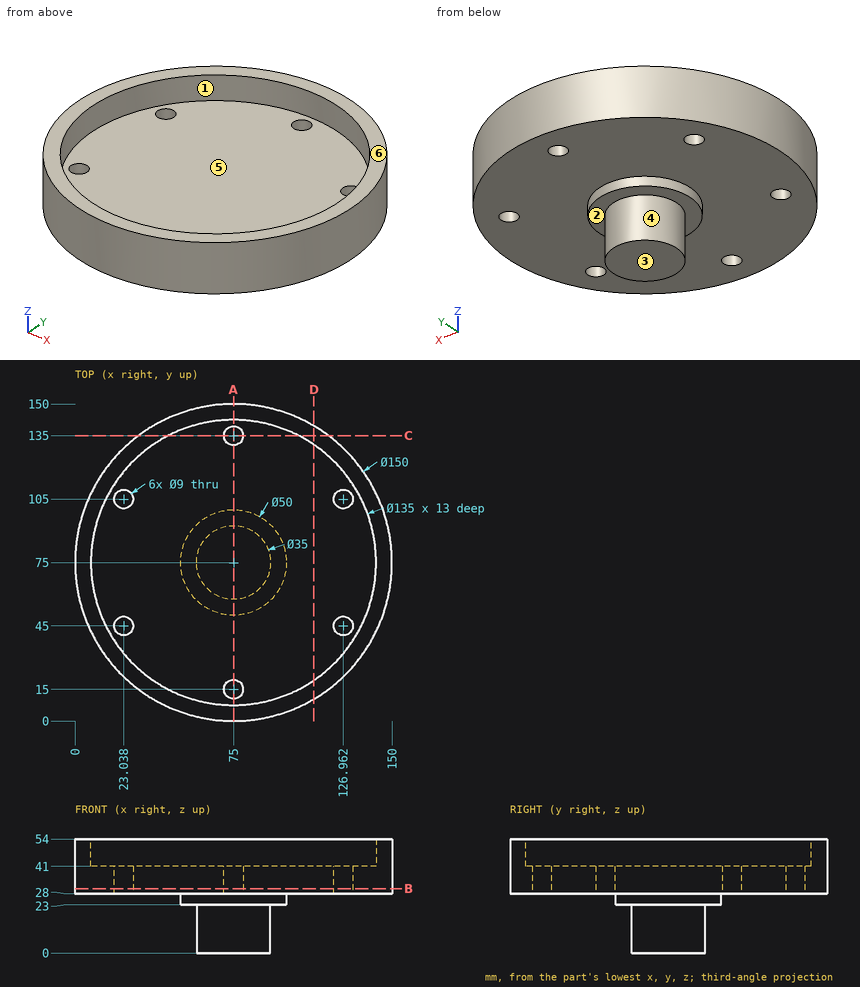
For this review, use the dimensioned drawing (mm, ordinates from the lowest corner) and the shaded views. A direction names the side the tool comes from. Round coordinates to 2 decimals unless told otherwise and drop trailing zeros. Order: outer loops, then holes, each group sorted by start corner. A loop starts at its lowest first (then second) coordinate and runs counter-clockwise, first axis right, second up. Notation, with made-up numbers: M 67,-2.5 L 116,-2.5 A26 ccw 116,36.5 Z; hole C 55.25,-20.5 d4. An arc over 180 degrees is marked long. Write each question's results on one line, items separated by ' | '. Start each with the question number.
1. Add section D-D (x = 113). State the section outline as (y, z) points.
2. Draft analysis for pull direction Y (two halves, no side actions). For the marked faces 4, 5 and 6, state which applies: pulls with the +Y half, pulls with the -Y half, needs draft (parallel to the pull), parting line crosses it, or undercut.
3. Clearance check with flat-ended pins moving along their axes: pin 1 Ø8 at (y, z) = (16.5, 29) entering from +X (1 decimal); pin 2 Ø8 at (x, y) = (23.04, 105) entering from -Z; pin 3 Ø3 at (x, z) = (74, 27) entering from -Y; pin 4 Ø12 at (x, z) = (98, 44.5) entering from +Y. State where each tip first meets the part, or that it passes through.
4. Add section C-C (y = 135). State the section outline as (x, z) points, then the cut area to 3 significant figures.
5. To check wall thickness, follow L1, parallel to Y at x = 75, z = 38; L2, parallel to Y at x = 75, z = 49.25; L3, parallel to Z at x = 110.5, y = 141. State the ranges of each line that lie inside material, in increasing order. Write a range as [from, to].
6. Add section A-A (x = 75). State the section outline as (y, z) points, then the cut area to 3 significant figures.
7. Tool access review of the marked faces 1, 2 and 3: name each direction out of +Z, -Z, +X, -X, +Y, -Y from which nothing blocks a thin tool from reaching the whole face with its end or side.
8. Add section B-B (z = 30.5). State the section outline as (x, y) points, then the cut area to 3 significant figures.
Output values:
1) outline: M 10.34,28 L 139.66,28 L 139.66,54 L 130.79,54 L 130.79,41 L 19.21,41 L 19.21,54 L 10.34,54 Z
2) face 4: parting line crosses it | face 5: undercut | face 6: needs draft
3) pin 1: x = 126.5 | pin 2: through | pin 3: y = 0 | pin 4: y = 148.05
4) outline: M 30,28 L 70.5,28 L 70.5,41 L 44.08,41 L 44.08,54 L 30,54 Z; M 79.5,28 L 120,28 L 120,54 L 105.92,54 L 105.92,41 L 79.5,41 Z | area: 1,420 mm^2
5) L1: [0, 10.5], [19.5, 130.5], [139.5, 150] | L2: [0, 7.5], [142.5, 150] | L3: [28, 54]
6) outline: M 0,28 L 10.5,28 L 10.5,41 L 7.5,41 L 7.5,54 L 0,54 Z; M 19.5,28 L 50,28 L 50,23 L 57.5,23 L 57.5,0 L 92.5,0 L 92.5,23 L 100,23 L 100,28 L 130.5,28 L 130.5,41 L 19.5,41 Z; M 139.5,28 L 150,28 L 150,54 L 142.5,54 L 142.5,41 L 139.5,41 Z | area: 2,970 mm^2
7) face 1: +Z | face 2: -Z | face 3: -Z, +X, -X, +Y, -Y
8) outline: C 75,75 d150; hole C 23.04,45 d9; hole C 23.04,105 d9; hole C 75,15 d9; hole C 75,135 d9; hole C 126.96,45 d9; hole C 126.96,105 d9 | area: 17,300 mm^2
